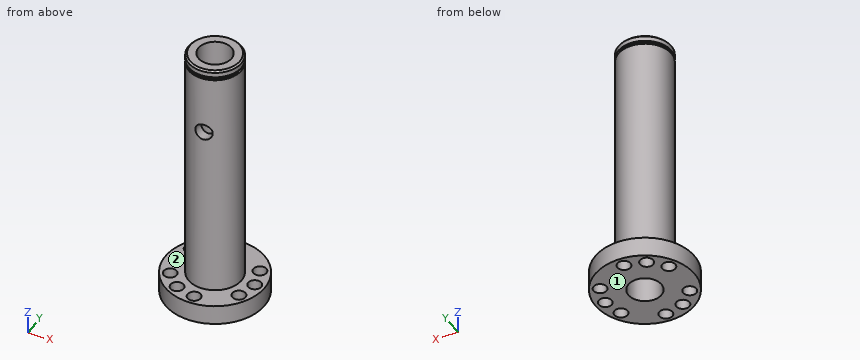
from build123d import *

# Parameters (mm, degrees)
SKETCH_1_R          = 15
SKETCH_1_R_2        = 2
SKETCH_1_R_3        = 5
EXTRUDE_1_DEPTH     = 10
SKETCH_2_R          = 8
SKETCH_2_R_2        = 5
EXTRUDE_2_DEPTH     = 70
SKETCH_3_R          = 2.5
CUT_EXTRUDE_1_DEPTH = 10
CUT_EXTRUDE_START   = -4
SKETCH_4_R          = 18.074037985
SKETCH_4_R_2        = 8
CUT_EXTRUDE_2_DEPTH = 4
SKETCH_5_W          = 0.5
SKETCH_5_H          = 1


with BuildPart() as part:
    # Sketch 1 → Extrude 1 (new body)
    with BuildSketch(Plane.XY):
        Circle(SKETCH_1_R)
        with Locations((0, 12)):
            Circle(SKETCH_1_R_2, mode=Mode.SUBTRACT)
        with Locations((10.392304845, 6)):
            Circle(SKETCH_1_R_2, mode=Mode.SUBTRACT)
        with Locations((10.392304845, -6)):
            Circle(SKETCH_1_R_2, mode=Mode.SUBTRACT)
        with Locations((0, -12)):
            Circle(SKETCH_1_R_2, mode=Mode.SUBTRACT)
        with Locations((-10.392304845, -6)):
            Circle(SKETCH_1_R_2, mode=Mode.SUBTRACT)
        with Locations((-10.392304845, 6)):
            Circle(SKETCH_1_R_2, mode=Mode.SUBTRACT)
        with Locations((-6, 10.392304845)):
            Circle(SKETCH_1_R_2, mode=Mode.SUBTRACT)
        with Locations((12, 0)):
            Circle(SKETCH_1_R_2, mode=Mode.SUBTRACT)
        with Locations((-6, -10.392304845)):
            Circle(SKETCH_1_R_2, mode=Mode.SUBTRACT)
        Circle(SKETCH_1_R_3, mode=Mode.SUBTRACT)
    extrude(amount=EXTRUDE_1_DEPTH)

    # Sketch 2 → Extrude 2 (add)
    with BuildSketch(Plane.XY.offset(10)):
        Circle(SKETCH_2_R)
        Circle(SKETCH_2_R_2, mode=Mode.SUBTRACT)
    extrude(amount=EXTRUDE_2_DEPTH)

    # Sketch 3 → Cut-Extrude 1 (cut)
    with BuildSketch(Plane(origin=(0, 0, 0), x_dir=(1, 0, 0), z_dir=(0, 1, 0))):
        with Locations(Location((0.676832819, -59, 0), (0, 0, 270))):
            Circle(SKETCH_3_R)
    extrude(amount=-CUT_EXTRUDE_1_DEPTH, mode=Mode.SUBTRACT)

    # Sketch 4 → Cut-Extrude 2 (cut)
    with BuildSketch(Plane.XY.offset(10).offset(CUT_EXTRUDE_START)):
        Circle(SKETCH_4_R)
        Circle(SKETCH_4_R_2, mode=Mode.SUBTRACT)
    extrude(amount=CUT_EXTRUDE_2_DEPTH, mode=Mode.SUBTRACT)

    # Fillet 1: read off the stored shape, not the designer's step
    # Fillet 1 outline → Fillet 1 (revolve, cut)
    with BuildSketch(Plane.XZ):
        Polygon((8, 80), (7.5, 80), (8, 79.5), align=None)
    revolve(axis=Axis((0, 0, 0), (0, 0, 1)), mode=Mode.SUBTRACT)

    # Sweep 2: sweep along a path in Sketch 6
    with BuildLine(Plane.XY.offset(80)) as sweep_2_path:
        CenterArc((0, 0), 7.5, 0, 360)
    # Sketch 5 → Sweep 2 (sweep, cut)
    with BuildSketch(Plane(origin=(0, 0, 0), x_dir=(1, 0, 0), z_dir=(0, 1, 0))):
        with Locations((7.75, -77.5)):
            Rectangle(SKETCH_5_W, SKETCH_5_H)
    sweep(path=sweep_2_path.line, mode=Mode.SUBTRACT)


solid = part.part
Geometry: final body of the model. Coordinates: model frame, mm. Face numbers are marked on the shaded views. A direction names the side the tool comes from. Round coordinates to 2 decimals unless told otherwise and drop trailing zeros. Order: outer loops, then holes, each group sorted by start corner. A loop starts at its lowest first (then second) coordinate and runs counter-clockwise, first axis right, second up.
Q1. Section D-D, the plane x = 11. Output: boundary loops of the cut face in (y, z).
Result sheet:
outline: (-10.2, 0) - (-7.91, 0) - (-7.91, 6) - (-10.2, 6) - close; (-4.09, 0) - (-1.73, 0) - (-1.73, 6) - (-4.09, 6) - close; (1.73, 0) - (4.09, 0) - (4.09, 6) - (1.73, 6) - close; (7.91, 0) - (10.2, 0) - (10.2, 6) - (7.91, 6) - close
Q2. Section C-C, the plane z = 52. Output: boundary loops of the cut face in (x, y), and give its area (3 significant figures).
Result sheet:
outline: circle Ø16 at (0, 0); hole circle Ø10 at (0, 0)
area: 123 mm2
Q3. Section A-A, the plane x = -10.75. Output: boundary loops of the cut face in (y, z), and give its area (3 significant figures).
Result sheet:
outline: (-10.46, 0) - (-7.97, 0) - (-7.97, 6) - (-10.46, 6) - close; (-4.03, 0) - (4.03, 0) - (4.03, 6) - (-4.03, 6) - close; (7.97, 0) - (10.46, 0) - (10.46, 6) - (7.97, 6) - close
area: 78.3 mm2
Q4. Material intervals for probe 1 along Y at (x, z) = (0, 2.25); probe 2 along Y at (x, z) = (-6, 3.15), sorted ascending.
Result sheet:
probe 1: y = -15 to -14, -10 to -5, 5 to 10, 14 to 15
probe 2: y = -13.75 to -12.39, -8.39 to 8.39, 12.39 to 13.75
Q5. Pin query (flat end, axial travel): pin 1 (3.5 mm diameter, centred on x = 10.39, y = 6, fed in from +Z); pin 2 (5 mm diameter, centred on x = 6.5, z = 22.5, fed in from -Y); pin 3 (4 mm diameter, centred on x = 5.5, z = 56, fed in from +Y); pin 4 (5 mm diameter, centred on x = 0, y = 12, fed in from +Z). Return the tip coordinate at first contact, or that it passes through.
Result sheet:
pin 1: passes through
pin 2: stops at y = -6.93
pin 3: stops at y = 7.19
pin 4: stops at z = 6
Q6. Section B-B, the plane y = 0. Give the number of separate pieces and of enclosed holes in the cut face, and give its area (3 significant figures).
Result sheet:
separate pieces: 3
enclosed holes: 0
area: 539 mm2
Q7. Access query for the marked faces 1 and 2. Directions: +Z, -Z, +X, -X, +Y, -Y. A direction counts if a zero-diameter tool reaches every point of the face in a straight line with its end or side. Return the directions, or none.
Result sheet:
face 1: -Z, +X, -X, +Y, -Y
face 2: +Z
